Geometry check sheet. Reference: drawing and pictorial views, mm from the part's lowest x, y, z. A direction names the side the tool comes from. Give positions to 0.01 mm unless a question says otherwise; leave off trailing zeros. Write each loop counter-clockwise with the first axis right and the second up, starting at its lowest first coordinate (ties: lowest second). Pieces come first, ordered by that corner, then holes. Notation, with made-up numbers: M -24,82 L -5,82 A23 ccw -5,117 Z; hole C 89,62 d2. An arc over 180 degrees is marked long. Answer as a JSON object with one key per item and string values.
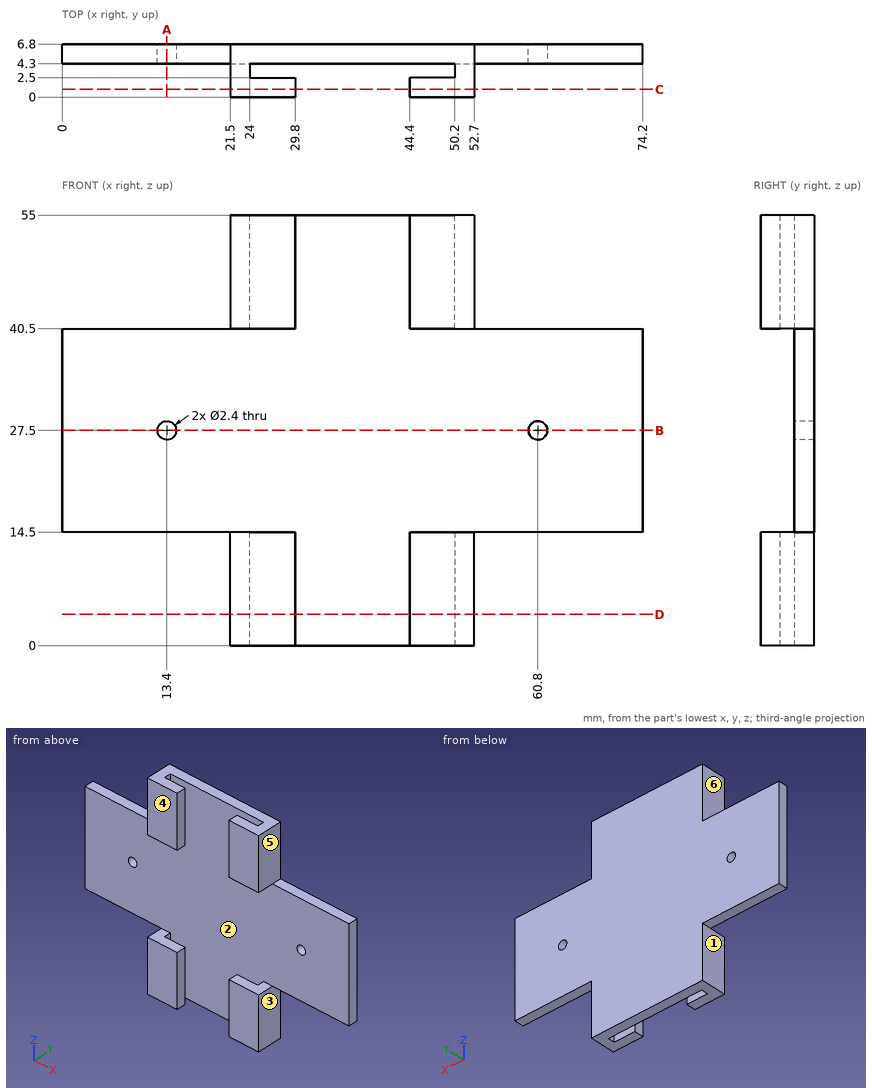
1) Section check D-D on z = 4. Record the boundary of the cut face in (x, y), and give its area (4 significant figures).
Completed:
{"outline": "M 21.5,0 L 29.8,0 L 29.8,2.5 L 24,2.5 L 24,4.3 L 50.2,4.3 L 50.2,2.5 L 44.4,2.5 L 44.4,0 L 52.7,0 L 52.7,6.8 L 21.5,6.8 Z", "area": "128.5 mm2"}
2) Release check for a two-part mould opening along X. For the marked faces 1, 2 and 3 record: pulls with the +X half, pulls with the -X half, needs draft (parallel to the pull), parting line crosses it, or undercut.
Completed:
{"face 1": "pulls with the -X half", "face 2": "undercut", "face 3": "pulls with the +X half"}
3) Access from +Z, -Z, +X, -X, +Y, -Y to the whole of each face (thin tool, end or side, straight path). Record for the marked faces 4, 5 and 6.
Completed:
{"face 4": "+Z, -Z, +X, -X, -Y", "face 5": "+Z, +X, +Y, -Y", "face 6": "+Z, -X, +Y, -Y"}
4) Section check B-B on z = 27.5. Record the boundary of the cut face in (x, y), and give its area (4 significant figures).
Completed:
{"outline": "M 0,4.3 L 12.2,4.3 L 12.2,6.8 L 0,6.8 Z; M 14.6,4.3 L 59.6,4.3 L 59.6,6.8 L 14.6,6.8 Z; M 62,4.3 L 74.2,4.3 L 74.2,6.8 L 62,6.8 Z", "area": "173.5 mm2"}
5) Section check A-A on x = 13.4. Record the boundary of the cut face in (y, z).
Completed:
{"outline": "M 4.3,14.5 L 6.8,14.5 L 6.8,26.3 L 4.3,26.3 Z; M 4.3,28.7 L 6.8,28.7 L 6.8,40.5 L 4.3,40.5 Z"}
6) Go/stop test with flat-tipped pins: pin 1 (0.8 mm diameter, centred on x = 13, y = 5.5, fed in from -Z); pin 2 (3 mm diameter, centred on y = 6, z = 47.5, fed in from +X); pin 3 (2 mm diameter, centred on x = 6, y = 6, fed in from +Z). Record where each tip stops, or that it passes through.
Completed:
{"pin 1": "stops at z = 14.5", "pin 2": "stops at x = 52.7", "pin 3": "stops at z = 40.5"}
7) Section check C-C on y = 1. Record the boundary of the cut face in (x, z), and give its area (3 significant figures).
Completed:
{"outline": "M 21.5,0 L 29.8,0 L 29.8,14.5 L 21.5,14.5 Z; M 21.5,40.5 L 29.8,40.5 L 29.8,55 L 21.5,55 Z; M 44.4,0 L 52.7,0 L 52.7,14.5 L 44.4,14.5 Z; M 44.4,40.5 L 52.7,40.5 L 52.7,55 L 44.4,55 Z", "area": "481 mm2"}
8) Thickness scan on L1, parallel to Z at x = 13.4, y = 5.45; L2, parallel to X at y = 2.25, z = 49; L3, parallel to Y at x = 45.5, z = 52. Record the ranges inside material, lowest first.
Completed:
{"L1": "z = 14.5 to 26.3, 28.7 to 40.5", "L2": "x = 21.5 to 29.8, 44.4 to 52.7", "L3": "y = 0 to 2.5, 4.3 to 6.8"}
